```python
from build123d import *

# Parameters (mm, degrees)
SKETCH_1_R      = 1.65
EXTRUDE_1_DEPTH = 15
EXTRUDE_2_DEPTH = 1.5


with BuildPart() as part:
    # 스케치1 → 보스-돌출1 (new body)
    with BuildSketch(Plane.XY):
        Circle(SKETCH_1_R)
    extrude(amount=EXTRUDE_1_DEPTH)

    # 스케치2 → 보스-돌출2 (add)
    with BuildSketch(Plane(origin=(0, 0, 15), x_dir=(-1, 0, 0), z_dir=(0, 0, -1))):
        Polygon((1.852010162, -2.435855433), (3.035517766, 0.385960132), (1.183507604, 2.821815565), (-1.852010162, 2.435855433), (-3.035517766, -0.385960132), (-1.183507604, -2.821815565), align=None)
    extrude(amount=-EXTRUDE_2_DEPTH)


solid = part.part
```
Here's how the part is built. I have some questions about the finished solid (model axes, mm). A direction names the side the tool comes from. Round coordinates to 2 decimals unless told otherwise and drop trailing zeros. Loops run counter-clockwise (first coordinate to the right, second up) from the corner with the lowest first, then second, coordinate; pieces in that order, holes last. Notation, with made-up numbers: (55, -14) -> (110, -14) arc R15 cw to (110, 4) -> close; hole circle Ø11 at (19.25, -3). An arc over 180 degrees is marked (long way). Answer as CSV lines item,"result". Start each with the question number.
1. Imagine slicing it at A-A on x = 0.5. Write out the boundary of the cut face in (y, z), plus the area to 3 significant figures.
2. I'm going to push flat-ended pins straight in: P1, Ø1.5, axis at y = 2, z = 12, coming from the -X side; P2, Ø1, axis at y = 1.5, z = 12.5, coming from the -X side. Where does each tip first touch, or does it pass through?
3. Imagine slicing it at B-B on z = 7.25. Write out the boundary of the cut face in (x, y), plus the area to 3 significant figures.
4. Imagine slicing it at D-D on y = 2.05. Write out the boundary of the cut face in (x, z).
5. For faces 1 (the face through (0, 0, 0)), 2 (the face through (0, -2, 15)), which set-ups out of +Z, -Z, +X, -X, +Y, -Y let a thin tool reach every point of the face, with its end or its side?
6. I need wall thicknesses on probe 1 along Z at (x, y) = (-1.25, 2.65); probe 2 along X at (y, z) = (-0.5, 1.25); probe 3 along X at (y, z) = (1.2, 15.5). Which ranges of each line are inside material? Lowest first, please. Write a range as from..to.
7. Imagine slicing it at C-C on y = 0.55. Write out the boundary of the cut face in (x, z), plus the area to 3 significant figures.
Solution:
1,outline,"(-2.73, 15) -> (-1.57, 15) -> (-1.57, 0) -> (1.57, 0) -> (1.57, 15) -> (2.61, 15) -> (2.61, 16.5) -> (-2.73, 16.5) -> close"
1,area,"55.2 mm²"
2,P1,"x = -1.08"
2,P2,"x = -1.31"
3,outline,"circle Ø3.3 at (0, 0)"
3,area,"8.55 mm²"
4,outline,"(-1.77, 15) -> (2.01, 15) -> (2.01, 16.5) -> (-1.77, 16.5) -> close"
5,face 1,"-Z, +X, -X, +Y, -Y"
5,face 2,"-Z"
6,probe 1,"15..16.5"
6,probe 2,"-1.57..1.57"
6,probe 3,"-2.42..2.37"
7,outline,"(-2.91, 15) -> (-1.56, 15) -> (-1.56, 0) -> (1.56, 0) -> (1.56, 15) -> (2.64, 15) -> (2.64, 16.5) -> (-2.91, 16.5) -> close"
7,area,"55.0 mm²"
